Model file for the job. Use its own axes, mm. A direction names the side the tool comes from. Coordinates: 2 decimals unless noted, no trailing zeros. Write each loop counter-clockwise with the first axis right and the second up, starting at its lowest first coordinate (ties: lowest second). Pieces come first, ordered by that corner, then holes. Notation, with made-up numbers: M 10.25,-34 L 26.25,-34 A17 ccw 26.25,-27 Z; hole C 68,7.5 d11. An arc over 180 degrees is marked long. One line per question, with ' | ' between items. Start each with the question number.
(1) Wall check: probe 1 along X at (y, z) = (-8, -2); probe 2 along Y at (x, z) = (27, -0.5); probe 3 along Y at (x, z) = (-22, -1.5). Give the ranges that are in metal, low to high.
(2) Cut at B-B (y = 33). Write the cut outline in (x, z) (1 decimal), plus the area to 3 significant figures.
(3) Cut at C-C (x = -1.5). Write the cut outline in (y, z) (1 decimal).
(4) Cut at A-A (z = -0.25). Write the cut outline in (x, y) (3 decimals), plus the area to 3 significant figures.
(5) Tool access for faces 1 (the face through (11, 1, 3.175)), 2 (the face through (4.83, -8.21, 0.04)): list every direction of +Z, -Z, +X, -X, +Y, -Y with a clear straight run to the whole face (end or side of a thin tool).
(6) Cut at D-D (y = -23). Write the cut outline in (x, z) (1 decimal), plus the area to 3 significant figures.
(7) Two-plate mould, pull along X, no slides. Class faces 3 (the face through (2.574, 43.727, 0.044)), 4 (the face through (11, 1, -3.175)), 5 (the face through (43.727, -2.574, 0.044)): +X half, -X half, draft (parallel to the pull), parting line (faces both ways), or undercut.
from build123d import *

# Parameters (mm, degrees)
BOSS_EXTRUDE1_DEPTH = 3.175


with BuildPart() as part:
    # Sketch2 → Boss-Extrude1 (new body, symmetric)
    with BuildSketch(Plane.XY):
        with BuildLine():
            ThreePointArc((-5.221965604, -36.452767418), (-4.196850428, -32.340432027), (0, -31.75))
            ThreePointArc((0, -31.75), (34.198681309, -29.952890094), (50.8, 0))
            Line((50.8, 0), (36.452767418, -5.221965604))
            ThreePointArc((36.452767418, -5.221965604), (32.340432027, -4.196850428), (31.75, 0))
            ThreePointArc((31.75, 0), (29.952890094, 34.198681309), (0, 50.8))
            Line((0, 50.8), (5.221965604, 36.452767418))
            ThreePointArc((5.221965604, 36.452767418), (4.196850428, 32.340432027), (0, 31.75))
            ThreePointArc((0, 31.75), (-34.198681309, 29.952890094), (-50.8, 0))
            Line((-50.8, 0), (-36.452767418, 5.221965604))
            ThreePointArc((-36.452767418, 5.221965604), (-32.340432027, 4.196850428), (-31.75, 0))
            ThreePointArc((-31.75, 0), (-29.952890094, -34.198681309), (0, -50.8))
            Line((0, -50.8), (-5.221965604, -36.452767418))
        make_face()
        Polygon((9.525, -5.499261314), (0, -10.998522628), (-9.525, -5.499261314), (-9.525, 5.499261314), (0, 10.998522628), (9.525, 5.499261314), align=None, mode=Mode.SUBTRACT)
    extrude(amount=BOSS_EXTRUDE1_DEPTH, both=True)


solid = part.part
Filled in:
1) probe 1: -34.52 to -5.19, 5.19 to 49.88 | probe 2: -33.39 to 38.25 | probe 3: -43.11 to 34.71
2) outline: M -28.1,-3.2 L -2.9,-3.2 L -2.9,3.2 L -28.1,3.2 Z; M 4.8,-3.2 L 30.7,-3.2 L 30.7,3.2 L 4.8,3.2 Z | area: 324 mm²
3) outline: M -50.8,-3.2 L -46.7,-3.2 L -46.7,3.2 L -50.8,3.2 Z; M -31.4,-3.2 L -10.1,-3.2 L -10.1,3.2 L -31.4,3.2 Z; M 10.1,-3.2 L 32.4,-3.2 L 32.4,3.2 L 10.1,3.2 Z
4) outline: M -50.8,0 L -36.453,5.222 A3.79 cw -31.75,0 A35.322 ccw 0,-50.8 L -5.222,-36.453 A3.79 cw 0,-31.75 A35.322 ccw 50.8,0 L 36.453,-5.222 A3.79 cw 31.75,0 A35.322 ccw 0,50.8 L 5.222,36.453 A3.79 cw 0,31.75 A35.322 ccw Z; hole M -9.525,-5.499 L 0,-10.999 L 9.525,-5.499 L 9.525,5.499 L 0,10.999 L -9.525,5.499 Z | area: 5,470 mm²
5) face 1: +Z, +X, -X, +Y, -Y | face 2: +Z, -Z
6) outline: M -34.5,-3.2 L 42.3,-3.2 L 42.3,3.2 L -34.5,3.2 Z | area: 488 mm²
7) face 3: -X half | face 4: draft | face 5: undercut
